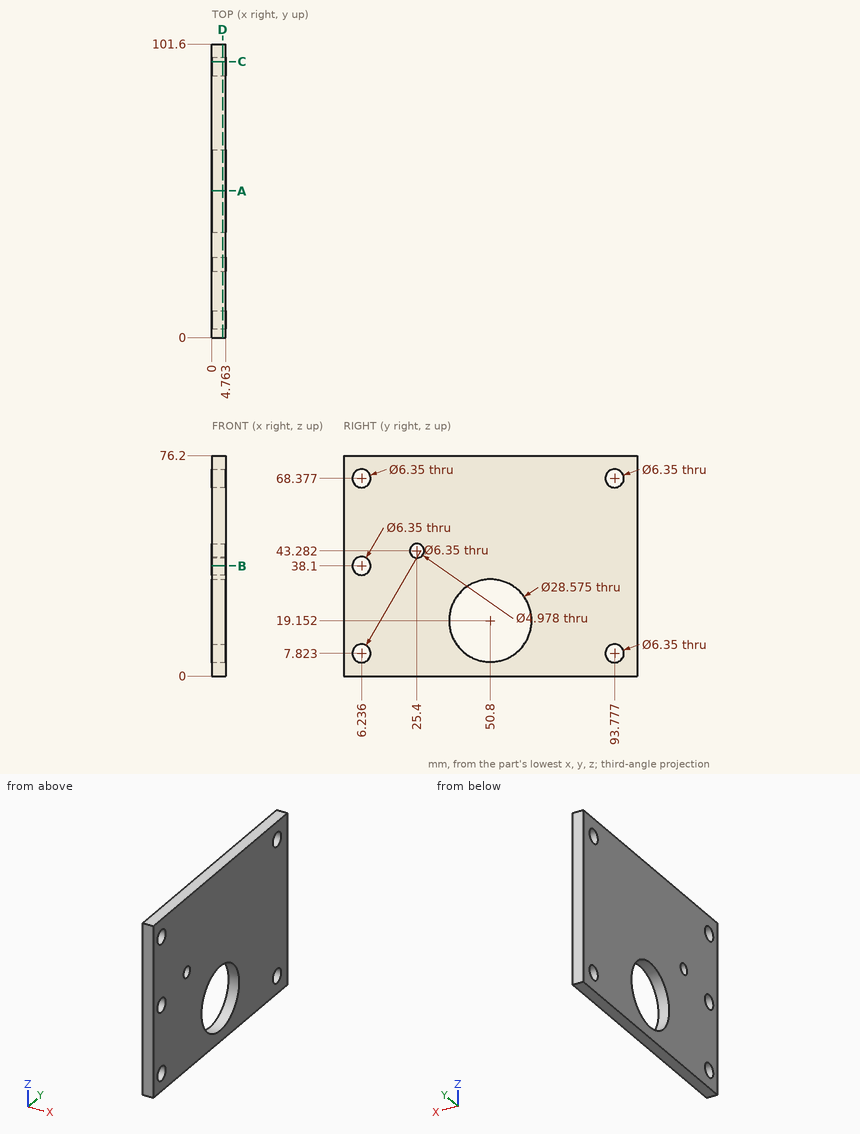
Part print with two shaded views. Sizes in mm from the minimum x, y, z corner. Coordinates: 2 decimals unless noted, no trailing zeros. Write each loop counter-clockwise with the first axis right and the second up, starting at its lowest first coordinate (ties: lowest second). Pieces come first, ordered by that corner, then holes.
1. Band-saw the part on C-C, the plane y = 95.5. Give the cut face in (x, z).
Answer block:
outline: (0, 0) - (4.76, 0) - (4.76, 5.16) - (0, 5.16) - close; (0, 10.49) - (4.76, 10.49) - (4.76, 65.71) - (0, 65.71) - close; (0, 71.04) - (4.76, 71.04) - (4.76, 76.2) - (0, 76.2) - close
2. Band-saw the part on B-B, the plane z = 38.1. Give the cut face in (x, y).
Answer block:
outline: (0, 0) - (4.76, 0) - (4.76, 3.06) - (0, 3.06) - close; (0, 9.41) - (4.76, 9.41) - (4.76, 101.6) - (0, 101.6) - close
3. Band-saw the part on A-A, the plane y = 50.8. Give the cut face in (x, z) (1 decimal).
Answer block:
outline: (0, 0) - (4.8, 0) - (4.8, 4.9) - (0, 4.9) - close; (0, 33.4) - (4.8, 33.4) - (4.8, 76.2) - (0, 76.2) - close
4. Drop a flat-ended pin along its axis: pin 1 (4 mm diameter, centred on y = 6.24, z = 68.38, fed in from -X) (3 decimals). Give the stop position or say it passes through.
Answer block:
pin 1: passes through
5. Drill centre lines: probe 1 along Y at (x, z) = (2.05, 38.1); probe 2 along Y at (x, z) = (1.2, 16) (1 decimal); probe 3 along Z at (x, y) = (4.5, 42) (1 decimal). Where is each one in solid material? Low to high.
Answer block:
probe 1: y = 0 to 3.06, 9.41 to 101.6
probe 2: y = 0 to 36.9, 64.7 to 101.6
probe 3: z = 0 to 7.9, 30.4 to 76.2
6. Band-saw the part on D-D, the plane x = 3.75. Give the number of separate pieces and of enclosed holes in the cut face, and give its area (3 significant figures).
Answer block:
separate pieces: 1
enclosed holes: 7
area: 6,920 mm2
